```python
from build123d import *

# Parameters (mm, degrees)
BOSS_EXTRUDE1_DEPTH              = 36
SKETCH2_R                        = 10.5
CUT_EXTRUDE1_DEPTH               = 74.681748079
SKETCH3_W                        = 28.5
SKETCH3_H                        = 29.5
CUT_EXTRUDE2_DEPTH               = 74.681748079
CHAMFER1_SIZE                    = 2
BOSS_EXTRUDE2_START              = -2
SKETCH6_R                        = 10.5
SKETCH6_R_2                      = 9
BOSS_EXTRUDE2_DEPTH              = 2
SKETCH10_R                       = 15
SKETCH10_R_2                     = 11
CUT_EXTRUDE4_DEPTH               = 0.6
SKETCH11_R                       = 12.5
CUT_EXTRUDE5_DEPTH               = 5
M2_5_CLEARANCE_HOLE1_D           = 2.9
M2_5_CLEARANCE_HOLE1_CSINK_D     = 2.95
M2_5_CLEARANCE_HOLE1_CSINK_ANGLE = 90
CUT_EXTRUDE6_DEPTH               = 74.681748079
CUT_EXTRUDE7_DEPTH               = 74.681748079


with BuildPart() as part:
    # Sketch1 → Boss-Extrude1 (new body)
    with BuildSketch(Plane.XY):
        Polygon((0, 0), (17, 0), (17, 29), (17, 62), (5, 62), (5, 22), (0, 22), align=None)
    extrude(amount=BOSS_EXTRUDE1_DEPTH)

    # Sketch2 → Cut-Extrude1 (cut, through all)
    with BuildSketch(Plane(origin=(17, 0, 0), x_dir=(0, 0, -1), z_dir=(1, 0, 0))):
        with Locations(Location((-18, 45, 0), (0, 0, 90))):
            Circle(SKETCH2_R)
    extrude(amount=-CUT_EXTRUDE1_DEPTH, mode=Mode.SUBTRACT)

    # Sketch3 → Cut-Extrude2 (cut, through all)
    with BuildSketch(Plane(origin=(17, 0, 0), x_dir=(0, 0, -1), z_dir=(1, 0, 0))):
        with Locations((-18, 14.75)):
            Rectangle(SKETCH3_W, SKETCH3_H)
    extrude(amount=-CUT_EXTRUDE2_DEPTH, mode=Mode.SUBTRACT)

    # Chamfer1
    chamfer1_edges = [part.edges().sort_by_distance(p)[0] for p in [
        (11, 29.5, 32.25),
        (11, 29.5, 3.75),
    ]]
    chamfer(chamfer1_edges, length=CHAMFER1_SIZE)

    # Sketch6 → Boss-Extrude2 (add)
    with BuildSketch(Plane.ZY.offset(-5).offset(BOSS_EXTRUDE2_START)):
        with Locations(Location((18, 45, 0), (0, 0, 90))):
            Circle(SKETCH6_R)
        with Locations(Location((18, 45, 0), (0, 0, 270))):
            Circle(SKETCH6_R_2, mode=Mode.SUBTRACT)
    extrude(amount=BOSS_EXTRUDE2_DEPTH)

    # Sketch10 → Cut-Extrude4 (cut)
    with BuildSketch(Plane.ZY.offset(-5)):
        with Locations(Location((18, 45, 0), (0, 0, 270))):
            Circle(SKETCH10_R)
        with Locations(Location((18, 45, 0), (0, 0, 270))):
            Circle(SKETCH10_R_2, mode=Mode.SUBTRACT)
    extrude(amount=-CUT_EXTRUDE4_DEPTH, mode=Mode.SUBTRACT)

    # Sketch11 → Cut-Extrude5 (cut)
    with BuildSketch(Plane(origin=(17, 0, 0), x_dir=(0, 0, -1), z_dir=(1, 0, 0))):
        with Locations((-18, 45)):
            Circle(SKETCH11_R)
    extrude(amount=-CUT_EXTRUDE5_DEPTH, mode=Mode.SUBTRACT)

    # M2.5 Clearance Hole1 (through all)
    with Locations(Plane.XY.offset(36)):
        with Locations((14.5, 13.75), (2.5, 13.75)):
            CounterSinkHole(M2_5_CLEARANCE_HOLE1_D / 2, M2_5_CLEARANCE_HOLE1_CSINK_D / 2, counter_sink_angle=M2_5_CLEARANCE_HOLE1_CSINK_ANGLE)

    # Sketch15 → Cut-Extrude6 (cut, through all)
    with BuildSketch(Plane(origin=(0, 0, 0), x_dir=(-1, 0, 0), z_dir=(0, 0, -1))):
        with BuildLine():
            Line((-13.05, 13.75), (-13.05, 7.75))
            ThreePointArc((-13.05, 7.75), (-14.5, 6.3), (-15.95, 7.75))
            Line((-15.95, 7.75), (-15.95, 13.75))
            ThreePointArc((-15.95, 13.75), (-14.5, 15.2), (-13.05, 13.75))
        make_face()
        with BuildLine():
            Line((-1.05, 13.75), (-1.05, 7.75))
            ThreePointArc((-1.05, 7.75), (-2.5, 6.3), (-3.95, 7.75))
            Line((-3.95, 7.75), (-3.95, 13.75))
            ThreePointArc((-3.95, 13.75), (-2.5, 15.2), (-1.05, 13.75))
        make_face()
    extrude(amount=-CUT_EXTRUDE6_DEPTH, mode=Mode.SUBTRACT)

    # Sketch17 → Cut-Extrude7 (cut, through all)
    with BuildSketch(Plane(origin=(17, 0, 0), x_dir=(0, 0, -1), z_dir=(1, 0, 0))):
        with BuildLine():
            Line((-23.916079783, 62), (-36, 62))
            Line((-36, 62), (-36, 45))
            ThreePointArc((-36, 45), (-32.671220742, 55.428580054), (-23.916079783, 62))
        make_face()
        with BuildLine():
            Line((0, 62), (-12.083920217, 62))
            ThreePointArc((-12.083920217, 62), (-3.328779258, 55.428580054), (0, 45))
            Line((0, 45), (0, 62))
        make_face()
    extrude(amount=-CUT_EXTRUDE7_DEPTH, mode=Mode.SUBTRACT)


solid = part.part
```
For this review, take the finished solid that the model builds, in its own axes (mm). A direction names the side the tool comes from. Round coordinates to 2 decimals unless told otherwise and drop trailing zeros. Loops run counter-clockwise (first coordinate to the right, second up) from the corner with the lowest first, then second, coordinate; pieces in that order, holes last.
(1) We need section A-A (x = 10.75). Give the boundary of the cut face in (y, z), plus the area to 3 significant figures.
Returned:
outline: (0, 0) - (45, 0) arc R18 ccw to (62, 12.08) - (62, 23.92) arc R18 ccw to (45, 36) - (0, 36) - (0, 32.25) - (27.5, 32.25) - (29.5, 30.25) - (29.5, 5.75) - (27.5, 3.75) - (0, 3.75) - close; hole circle Ø21 at (45, 18)
area: 938 mm2
(2) We need section C-C (z = 13). Give the boundary of the cut face in (x, y), plus the area to 3 significant figures.
Returned:
outline: (5, 29.5) - (17, 29.5) - (17, 33.54) - (12, 33.54) - (12, 35.77) - (7, 35.77) - (7, 37.52) - (5, 37.52) - (5, 35.2) - (5.6, 35.2) - (5.6, 30.86) - (5, 30.86) - close; (5, 52.48) - (7, 52.48) - (7, 54.23) - (12, 54.23) - (12, 56.46) - (17, 56.46) - (17, 62) - (5, 62) - (5, 59.14) - (5.6, 59.14) - (5.6, 54.8) - (5, 54.8) - close
area: 148 mm2
(3) Mouldability with a two-part tool opening along Z and no side actions: class faces 1 (the cylindrical face through (14.535, 37.394, 27.92)), 2 (the cylindrical face through (11.08, 55.3, 32.76)), 3 (the flat face through (13.05, 11, 34)) as released by +Z, released by -Z, zero draft, split by the parting line, or undercut.
Returned:
face 1: undercut
face 2: released by +Z
face 3: zero draft
(4) Wall thickness on line 1 along Z through (x, y) = (1.25, 15); line 2 along Z through (x, y) = (5.3, 45); line 3 along Z through (x, y) = (5.65, 45): over which ranges is each line inside the solid? List them lowest first.
Returned:
line 1: z = 0 to 3.75, 32.25 to 36
line 2: z = 0 to 3, 7 to 9, 27 to 29, 33 to 36
line 3: z = 0 to 9, 27 to 36
(5) We need section D-D (y = 26). Give the boundary of the cut face in (x, z).
Returned:
outline: (5, 0) - (17, 0) - (17, 3.75) - (5, 3.75) - close; (5, 32.25) - (17, 32.25) - (17, 36) - (5, 36) - close
(6) Tool access review of faces 4 (the flat face through (8, 0, 34)), 5 (the flat face through (11.08, 28.51, 4.76)), 6 (the cylindrical face through (5.296, 59.985, 18.66)), 7 (the flat face through (15.95, 11, 34)), 8 (the cylindrical face through (6, 54, 18)): name each direction out of +Z, -Z, +X, -X, +Y, -Y from which nothing blocks a thin tool from reaching the whole face with its end or side.
Returned:
face 4: +Z, -Z, +X, -X, -Y
face 5: +X, -X, -Y
face 6: -X
face 7: +Z, -Z
face 8: +X, -X
(7) Clearance check with flat-ended pins moving along their axes: P1, Ø1.5, axis at x = 10.5, y = 50.5, coming from the -Z side; P2, Ø15, axis at y = 39.5, z = 22, coming from the -X side; P3, Ø1, axis at y = 6.5, z = 31.5, coming from the -X side; P4, Ø5, axis at x = 11.5, z = 24.5, coming from the -Y side. State where each tip first meets the part, or that it passes through.
Returned:
P1: stops at z = 0.64
P2: stops at x = 5
P3: passes through
P4: stops at y = 29.5
(8) We need section B-B (x = 2.5). Give the boundary of the cut face in (y, z) (3 decimals), plus the area to 3 significant figures.
Returned:
outline: (0, 0) - (6.3, 0) - (6.3, 3.75) - (0, 3.75) - close; (0, 32.25) - (6.3, 32.25) - (6.3, 36) - (0, 36) - close; (15.2, 0) - (22, 0) - (22, 3.75) - (15.2, 3.75) - close; (15.2, 32.25) - (22, 32.25) - (22, 36) - (15.225, 36) - (15.2, 35.975) - close
area: 98.2 mm2
